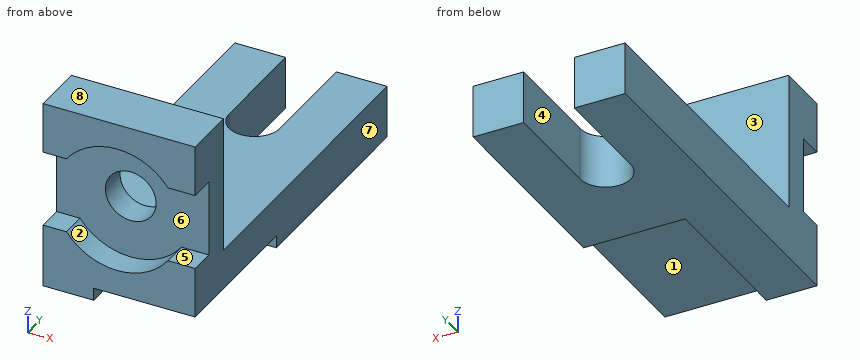
Autodesk Fusion 360 part; units mm, degrees
sketch "Sketch1" plane through (0, 0, 0) normal (0, 1, 0) x (1, 0, 0)
  line L0 (-35.1053, -42) -> (36.8947, -42)
  line L1 (36.8947, -42) -> (36.8947, 48)
  line L2 (36.8947, 48) -> (-35.1053, 48)
  line L3 (-35.1053, 48) -> (-35.1053, -42)
  point P0 (0.8947, 48)
  dimension "d3" = 90
  dimension "d4" = 72
  dimension "d7" = 48
extrude "Extrude1" add sketch "Sketch1" along normal blind 25
sketch "Sketch2" plane through (0, 0, 0) normal (0, -1, 0) x (1, 0, 0)
  line L0 (-35.1053, 42) -> (-35.1053, -48)
  line L1 (-35.1053, -48) -> (36.8947, -48)
  line L2 (36.8947, -48) -> (36.8947, 42)
  line L3 (36.8947, 42) -> (-35.1053, 42)
  line L4 (-35.1053, -18) -> (-24, -18)
  line L5 (24, -18) -> (36.8947, -18)
  line L6 (24, 18) -> (36.8947, 18)
  line L7 (-24, 18) -> (-35.1053, 18)
  arc A0 (-24, -18) -> (24, -18) centre (0, 0) ccw
  arc A1 (24, 18) -> (-24, 18) centre (0, 0) ccw
  dimension "d11" = 60
  dimension "d12" = 30
  dimension "d13" = 36
extrude "Extrude2" cut sketch "Sketch2" against normal blind 12 contours L0 L2 L4 L5 L6 L7 A0 A1
sketch "Sketch3" plane through (0, 12, 0) normal (0, -1, 0) x (1, 0, 0)
  arc A0 (24, 18) -> (-24, 18) centre (0, 0) ccw
  line L0 (-24, 18) -> (-35.1053, 18)
  line L1 (-35.1053, 18) -> (-35.1053, -18)
  line L2 (-35.1053, -18) -> (-24, -18)
  arc A1 (-24, -18) -> (24, -18) centre (0, 0) ccw
  line L3 (24, -18) -> (36.8947, -18)
  line L4 (36.8947, -18) -> (36.8947, 18)
  line L5 (36.8947, 18) -> (24, 18)
  circle A2 centre (0, 0) radius 12
  dimension "d16" = 24
extrude "Extrude3" cut sketch "Sketch3" against normal blind 13 contours A2
sketch "Sketch4" plane through (0, 25, 0) normal (0, 1, 0) x (-1, 0, 0)
  circle A0 centre (0, 0) radius 12
  line L0 (35.1053, -48) -> (35.1053, 42)
  line L1 (35.1053, 42) -> (-36.8947, 42)
  line L2 (-36.8947, 42) -> (-36.8947, -48)
  line L3 (-36.8947, -48) -> (35.1053, -48)
  line L4 (-36.8947, -48) -> (35.1053, -48)
  line L5 (35.1053, -48) -> (35.1053, -23)
  line L6 (35.1053, -23) -> (-36.8947, -23)
  line L7 (-36.8947, -23) -> (-36.8947, -48)
  dimension "d19" = 25
extrude "Extrude4" add sketch "Sketch4" along normal blind 145 contours L0 L2 L3 L4 L5 L6 L7
sketch "Sketch5" plane through (0, 0, -23) normal (0, 0, 1) x (-1, 0, 0)
  line L0 (35.1053, -25) -> (-36.8947, -25)
  line L1 (-36.8947, -25) -> (-36.8947, -170)
  line L2 (-36.8947, -170) -> (35.1053, -170)
  line L3 (35.1053, -170) -> (35.1053, -25)
  line L4 (11.1053, -170) -> (11.1053, -120)
  arc A0 (11.1053, -120) -> (-12.8947, -120) centre (-0.8947, -120) ccw
  line L5 (-12.8947, -120) -> (-12.8947, -170)
  line L6 (11.1053, -170) -> (-12.8947, -170)
  dimension "d22" = 24
  dimension "d23" = 24
  dimension "d24" = 50
extrude "Extrude5" cut sketch "Sketch5" against normal blind 25 contours L2 L4 A0 L5 L6
sketch "Sketch6" plane through (0, 0, -48) normal (0, 0, -1) x (1, 0, 0)
  line L0 (-11.1053, -170) -> (-11.1053, -120)
  arc A0 (12.8947, -120) -> (-11.1053, -120) centre (0.8947, -120) ccw
  line L1 (12.8947, -120) -> (12.8947, -170)
  line L2 (12.8947, -170) -> (36.8947, -170)
  line L3 (36.8947, -170) -> (36.8947, 0)
  line L4 (36.8947, 0) -> (-35.1053, 0)
  line L5 (-35.1053, 0) -> (-35.1053, -170)
  line L6 (-35.1053, -170) -> (-11.1053, -170)
  line L7 (36.8947, 0) -> (-11.1053, 0)
  line L8 (-11.1053, 0) -> (-11.1053, -72)
  line L9 (-11.1053, -72) -> (36.8947, -72)
  line L10 (36.8947, -72) -> (36.8947, 0)
  dimension "d27" = 48
  dimension "d28" = 72
extrude "Extrude6" cut sketch "Sketch6" against normal blind 6 contours L3 L4 L7 L8 L9 L10
Geometry: final body of the model. Coordinates: model frame, mm. Face numbers are marked on the shaded views. A direction names the side the tool comes from. Coordinates: 2 decimals unless noted, no trailing zeros. Order: outer loops, then holes, each group sorted by start corner. A loop starts at its lowest first (then second) coordinate and runs counter-clockwise, first axis right, second up.
Item 1: Section query C-C (y = 153). Output: boundary loops of the cut face in (x, z).
Answer:
outline: (-35.11, -48) - (-11.11, -48) - (-11.11, -23) - (-35.11, -23) - close; (12.89, -48) - (36.89, -48) - (36.89, -23) - (12.89, -23) - close
Item 2: Section query D-D (y = 48). Output: boundary loops of the cut face in (x, z).
Answer:
outline: (-35.11, -48) - (-11.11, -48) - (-11.11, -42) - (36.89, -42) - (36.89, -23) - (-35.11, -23) - close
Item 3: Section query A-A (z = 0). Output: boundary loops of the cut face in (x, y).
Answer:
outline: (-35.11, 12) - (-12, 12) - (-12, 25) - (-35.11, 25) - close; (12, 12) - (36.89, 12) - (36.89, 25) - (12, 25) - close
Item 4: Draft query along Z for the marked faces 6, 7 and 8. Return one class per face: released by +Z, released by -Z, zero draft, split by the parting line, or undercut.
Answer:
face 6: undercut
face 7: zero draft
face 8: released by +Z
Item 5: Material intervals for line 1 along Z through (x, y) = (-18, 8); line 2 along Z through (x, y) = (0, 20); line 3 along Z through (x, y) = (3, 90), sorted ascending.
Answer:
line 1: z = -48 to -24, 24 to 42
line 2: z = -42 to -12, 12 to 42
line 3: z = -48 to -23
Item 6: Section query B-B (x = 0). Output: boundary loops of the cut face in (y, z), then the cut area to 3 significant figures.
Answer:
outline: (0, -42) - (72, -42) - (72, -48) - (108.03, -48) - (108.03, -23) - (25, -23) - (25, -12) - (12, -12) - (12, -30) - (0, -30) - close; (0, 30) - (12, 30) - (12, 12) - (25, 12) - (25, 42) - (0, 42) - close
area: 2,860 mm2
Item 7: Access query for the marked faces 1, 2, 3, 4 and 5. Directions: +Z, -Z, +X, -X, +Y, -Y. A direction counts if a zero-diameter tool reaches every point of the face in a straight line with its end or side. Return the directions, or none.
Answer:
face 1: -Z, +X, -Y
face 2: -Y
face 3: +Z, +X, -X, +Y
face 4: +Z, -Z, +Y
face 5: +X, -X, -Y
Item 8: Contact query for flat-ended pins moving along their axis: P1, Ø1.8, axis at y = 48.5, z = -45.5, coming from the +X side; P2, Ø12, axis at x = 28, y = 30, coming from the -Z side; P3, Ø6.5, axis at x = 22.5, z = -45.5, coming from the -Y side. Output: stop coordinate, or through.
Answer:
P1: stops at x = -11.11
P2: stops at z = -42
P3: stops at y = 72
